```python
from build123d import *

# Parameters (mm, degrees)
SKETCH_2_R      = 14.5
EXTRUDE_1_DEPTH = 14
SKETCH_3_R      = 11
EXTRUDE_2_DEPTH = 49
FILLET_1_R      = 1


with BuildPart() as part:
    # 草图2 → 凸台-拉伸1 (new body)
    with BuildSketch(Plane(origin=(0, 0, 0), x_dir=(1, 0, 0), z_dir=(0, 1, 0))):
        with Locations(Location((0, 0, 0), (0, 0, 270))):
            Circle(SKETCH_2_R)
    extrude(amount=EXTRUDE_1_DEPTH)

    # 草图3 → 凸台-拉伸2 (add)
    with BuildSketch(Plane.XZ):
        with Locations(Location((0, 0, 0), (0, 0, 90))):
            Circle(SKETCH_3_R)
    extrude(amount=EXTRUDE_2_DEPTH)

    # 圆角1
    fillet_1_edges = [part.edges().sort_by_distance(p)[0] for p in [
        (0, 14, -14.5),
    ]]
    fillet(fillet_1_edges, radius=FILLET_1_R)


solid = part.part
```
Check sheet for the modelled part. Datum: model origin and axes. Units: mm. A direction names the side the tool comes from. Round coordinates to 2 decimals unless told otherwise and drop trailing zeros. Order: outer loops, then holes, each group sorted by start corner. A loop starts at its lowest first (then second) coordinate and runs counter-clockwise, first axis right, second up. Notation, with made-up numbers: (18, -15) - (54, -15) arc R13 cw to (54, 7) - close; hole circle Ø4 at (-10.75, 36.5). An arc over 180 degrees is marked (long way). Write item = value, one per line.
Q1. Go/stop test with flat-tipped pins: pin 1 (3 mm diameter, centred on x = -7.5, y = -42.5, fed in from -Z); pin 2 (3 mm diameter, centred on x = 9, z = -11, fed in from -Y); pin 3 (8 mm diameter, centred on x = 11, y = 7, fed in from +Z). Record where each tip stops, or that it passes through.
Computed:
pin_1 = -9.22
pin_2 = 0
pin_3 = 12.7
Q2. Thickness scan on line 1 along Y through (x, z) = (-3, 12.5); line 2 along X through (y, z) = (9.5, 3); line 3 along X through (y, z) = (-41.5, -8). Record the ranges inside material, lowest first.
Computed:
line_1 = 0 to 14
line_2 = -14.19 to 14.19
line_3 = -7.55 to 7.55
Q3. Section check B-B (x = 0). Record the boundary of the cut face in (y, z), and give its area (3 significant figures).
Computed:
outline = (-49, -11) - (0, -11) - (0, -14.5) - (13, -14.5) arc R1 ccw to (14, -13.5) - (14, 13.5) arc R1 ccw to (13, 14.5) - (0, 14.5) - (0, 11) - (-49, 11) - close
area = 1,480 mm^2
Q4. Section check A-A (z = 0). Record the boundary of the cut face in (x, y), and give its area (3 significant figures).
Computed:
outline = (-14.5, 0) - (-11, 0) - (-11, -49) - (11, -49) - (11, 0) - (14.5, 0) - (14.5, 13) arc R1 ccw to (13.5, 14) - (-13.5, 14) arc R1 ccw to (-14.5, 13) - close
area = 1,480 mm^2
Q5. Tool access check on faces 1 (the face through (10.74, -24.16, -2.38)), 2 (the face through (-5.554, 6.409, 13.394)). Record the directions out of +Z, -Z, +X, -X, +Y, -Y that give a thin tool (end or side, any length) a straight path to the whole face; none if there is none.
Computed:
face_1 = -Y
face_2 = +Y, -Y
Q6. Section check C-C (y = -18.5). Record the boundary of the cut face in (x, z), and give its area (3 significant figures).
Computed:
outline = circle Ø22 at (0, 0)
area = 380 mm^2
Q7. Section check D-D (y = 4). Record the boundary of the cut face in (x, z), and give its area (3 significant figures).
Computed:
outline = circle Ø29 at (0, 0)
area = 661 mm^2
